Source: CAD feature listing. Evaluate the final solid. Frame: model axes, mm. Face numbers are marked on the shaded views. A direction names the side the tool comes from. Round coordinates to 2 decimals unless told otherwise and drop trailing zeros. Order: outer loops, then holes, each group sorted by start corner. A loop starts at its lowest first (then second) coordinate and runs counter-clockwise, first axis right, second up. Notation, with made-up numbers: (12, -25) -> (33, -25) arc R27 cw to (33, 6) -> close; hole circle Ø6 at (6.5, 45.5). An arc over 180 degrees is marked (long way). Answer as CSV lines item,"result".
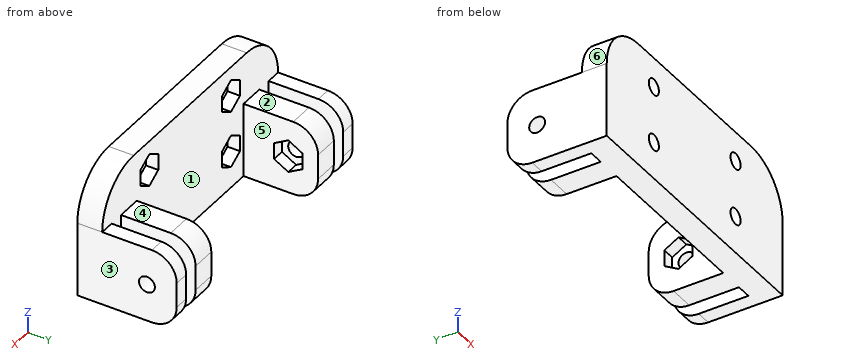
from build123d import *

# Parameters (mm, degrees)
F1_DEPTH  = 15
F2_R      = 1.6
F3_DEPTH  = 56.001
F5_DEPTH  = 2.5
F7_DEPTH  = 2.5
F8_W      = 56
F8_H      = 5
F9_DEPTH  = 10
F10_R     = 1.6
F11_DEPTH = 5.001
F13_DEPTH = 2.5
F14_R     = 10
F15_R     = 5


with BuildPart() as f1:
    # F0 (on Top) → F1 (new body)
    with BuildSketch(Plane.XY):
        Polygon((-28, 20), (-28, 0), (28, 0), (28, 20), (25, 20), (25, 5), (22, 5), (22, 20), (17, 20), (17, 5), (-17, 5), (-17, 20), (-22, 20), (-22, 5), (-25, 5), (-25, 20), align=None)
    extrude(amount=F1_DEPTH)

    # F2 (on face) → F3 (cut, through all)
    with BuildSketch(Plane(origin=(-28, 0, 0), x_dir=(0, -1, 0), z_dir=(-1, 0, 0))):
        with Locations((-14, 7.5)):
            Circle(F2_R)
    extrude(amount=-F3_DEPTH, mode=Mode.SUBTRACT)

    # F4 (on face) → F5 (cut)
    with BuildSketch(Plane.YZ.offset(-17)):
        Polygon((16.85, 5.854552), (16.85, 9.145448), (14, 10.790897), (11.15, 9.145448), (11.15, 5.854552), (14, 4.209103), align=None)
    extrude(amount=-F5_DEPTH, mode=Mode.SUBTRACT)

    # F6 (on face) → F7 (cut)
    with BuildSketch(Plane(origin=(17, 0, 0), x_dir=(0, -1, 0), z_dir=(-1, 0, 0))):
        Polygon((-11.15, 5.854552), (-11.15, 9.145448), (-14, 10.790897), (-16.85, 9.145448), (-16.85, 5.854552), (-14, 4.209103), align=None)
    extrude(amount=-F7_DEPTH, mode=Mode.SUBTRACT)

    # F8 (on face) → F9 (join)
    with BuildSketch(Plane.XY.offset(15)):
        with Locations((0, 2.5)):
            Rectangle(F8_W, F8_H)
    extrude(amount=F9_DEPTH)

    # F10 (on face) → F11 (cut, through all)
    with BuildSketch(Plane(origin=(0, 5, 0), x_dir=(-1, 0, 0), z_dir=(0, 1, 0))):
        with Locations((-13, 7.5)):
            Circle(F10_R)
        with Locations((13, 7.5)):
            Circle(F10_R)
        with Locations((-13, 19)):
            Circle(F10_R)
        with Locations((13, 19)):
            Circle(F10_R)
    extrude(amount=-F11_DEPTH, mode=Mode.SUBTRACT)

    # F12 (on face) → F13 (cut)
    with BuildSketch(Plane(origin=(0, 5, 0), x_dir=(-1, 0, 0), z_dir=(0, 1, 0))):
        Polygon((-10.15, 5.854552), (-10.15, 9.145448), (-13, 10.790897), (-15.85, 9.145448), (-15.85, 5.854552), (-13, 4.209103), align=None)
        Polygon((10.15, 9.145448), (10.15, 5.854552), (13, 4.209103), (15.85, 5.854552), (15.85, 9.145448), (13, 10.790897), align=None)
        Polygon((-15.85, 20.645448), (-15.85, 17.354552), (-13, 15.709103), (-10.15, 17.354552), (-10.15, 20.645448), (-13, 22.290897), align=None)
        Polygon((15.85, 17.354552), (15.85, 20.645448), (13, 22.290897), (10.15, 20.645448), (10.15, 17.354552), (13, 15.709103), align=None)
    extrude(amount=-F13_DEPTH, mode=Mode.SUBTRACT)

    # F14
    f14_edges = [f1.edges().sort_by_distance(p)[0] for p in [
        (28, 2.5, 25),
        (-28, 2.5, 25),
    ]]
    fillet(f14_edges, radius=F14_R)

    # F15
    f15_edges = [f1.edges().sort_by_distance(p)[0] for p in [
        (26.5, 20, 15),
        (19.5, 20, 15),
        (26.5, 20, 0),
        (19.5, 20, 0),
        (-19.5, 20, 0),
        (-26.5, 20, 0),
        (-26.5, 20, 15),
        (-19.5, 20, 15),
    ]]
    fillet(f15_edges, radius=F15_R)


solid = f1.part
1. Section query A-A on z = 18. Return loops of the section in (x, y), and give its area (3 significant figures).
Results below:
outline,"(-27.54, 0) -> (-14.25, 0) -> (-14.25, 2.5) -> (-15.85, 2.5) -> (-15.85, 5) -> (-27.54, 5) -> close; (-11.75, 0) -> (11.75, 0) -> (11.75, 2.5) -> (10.15, 2.5) -> (10.15, 5) -> (-10.15, 5) -> (-10.15, 2.5) -> (-11.75, 2.5) -> close; (14.25, 0) -> (27.54, 0) -> (27.54, 5) -> (15.85, 5) -> (15.85, 2.5) -> (14.25, 2.5) -> close"
area,"234 mm2"
2. Reachability of the marked faces 4, 5 and 6 from +Z, -Z, +X, -X, +Y, -Y: full face, straight path, thin tool, end or side. Return the list, or none.
Results below:
face 4,"+Z, +X, -X, +Y"
face 5,"+Z, -Z, +Y"
face 6,"+Z, -X, +Y, -Y"
3. Line query: L1, parallel to X at y = 4, z = 8; L2, parallel to Z at x = -13, y = 1.1; L3, parallel to X at y = 16.75, z = 8.5. Output: solid intervals per line, ascending. Write a range as [from, to].
Results below:
L1,"[-28, -15.85], [-10.15, 10.15], [15.85, 28]"
L2,"[0, 5.9], [9.1, 17.4], [20.6, 25]"
L3,"[-28, -25], [-22, -19.5], [19.5, 22], [25, 28]"
4. Section query D-D on x = 1. Return loops of the section in (y, z).
Results below:
outline,"(0, 0) -> (5, 0) -> (5, 25) -> (0, 25) -> close"
5. Section query B-B on y = 4.25. Give the number of separate pieces and of enclosed holes in the cut face, and give its area (3 significant figures).
Results below:
separate pieces,"1"
enclosed holes,"4"
area,"1,240 mm2"
6. Mould query, pull axis X, two halves, no side actions, for the marked faces 1, 2 and 3. Classes: released by +X, released by -X, zero draft, split by the parting line, or undercut.
Results below:
face 1,"undercut"
face 2,"zero draft"
face 3,"released by +X"
7. Section query C-C on z = 13.5. Return loops of the section in (x, y).
Results below:
outline,"(-28, 0) -> (28, 0) -> (28, 18.57) -> (25, 18.57) -> (25, 5) -> (22, 5) -> (22, 18.57) -> (17, 18.57) -> (17, 5) -> (-17, 5) -> (-17, 18.57) -> (-22, 18.57) -> (-22, 5) -> (-25, 5) -> (-25, 18.57) -> (-28, 18.57) -> close"
8. Pin query (flat end, axial travel): pin 1 (3 mm diameter, centred on x = 14, z = 8, fed in from +Y); pin 2 (3 mm diameter, centred on x = -15, z = 21, fed in from +Y); pin 3 (2 mm diameter, centred on y = 4, z = 18, fed in from +X). Return the tip coordinate at first contact, or that it passes through.
Results below:
pin 1,"y = 2.5"
pin 2,"y = 5"
pin 3,"x = 27.8"
